Could you check a few things on this model? Use its own coordinates, in mm. Face numbers are marked on the shaded views. Give positions to 0.01 mm unless a question says otherwise; leave off trailing zeros. Order: outer loops, then holes, each group sorted by start corner. A loop starts at its lowest first (then second) coordinate and runs counter-clockwise, first axis right, second up. Notation, with made-up numbers: M -38,-15 L 15,-15 A18 ccw 15,8 Z; hole C -14,32 d8. An arc over 180 degrees is marked long. Answer in a Markdown table with one row per item. Add a question column.
```python
from build123d import *

# Parameters (mm, degrees)
F0_R     = 50
F0_R_2   = 8.25
F1_DEPTH = 22
F2_R     = 55
F3_DEPTH = 3


with BuildPart() as f1:
    # F0 (on Top) → F1 (new body)
    with BuildSketch(Plane.XY):
        Circle(F0_R)
        with BuildLine():
            Line((-33.445853, -33.728696), (-7.458661, -7.741504))
            ThreePointArc((-7.458661, -7.741504), (-5.97238, -8.938298), (-4.297911, -9.853449))
            Line((-4.297911, -9.853449), (-18.362078, -43.807352))
            ThreePointArc((-18.362078, -43.807352), (-26.389586, -39.494807), (-33.445853, -33.728696))
        make_face(mode=Mode.SUBTRACT)
        with BuildLine():
            ThreePointArc((-3.928359, -10.006523), (-2.097221, -10.543442), (-0.2, -10.748139))
            Line((-0.2, -10.748139), (-0.2, -47.499579))
            ThreePointArc((-0.2, -47.499579), (-9.26679, -46.587301), (-17.992526, -43.960425))
            Line((-17.992526, -43.960425), (-3.928359, -10.006523))
        make_face(mode=Mode.SUBTRACT)
        with BuildLine():
            ThreePointArc((-9.853449, -4.297911), (-8.938298, -5.97238), (-7.741504, -7.458661))
            Line((-7.741504, -7.458661), (-33.728696, -33.445853))
            ThreePointArc((-33.728696, -33.445853), (-39.494807, -26.389586), (-43.807352, -18.362078))
            Line((-43.807352, -18.362078), (-9.853449, -4.297911))
        make_face(mode=Mode.SUBTRACT)
        with BuildLine():
            Line((-47.499579, -0.2), (-10.748139, -0.2))
            ThreePointArc((-10.748139, -0.2), (-10.543442, -2.097221), (-10.006523, -3.928359))
            Line((-10.006523, -3.928359), (-43.960425, -17.992526))
            ThreePointArc((-43.960425, -17.992526), (-46.587301, -9.26679), (-47.499579, -0.2))
        make_face(mode=Mode.SUBTRACT)
        with BuildLine():
            Line((0.2, -47.499579), (0.2, -10.748139))
            ThreePointArc((0.2, -10.748139), (2.097221, -10.543442), (3.928359, -10.006523))
            Line((3.928359, -10.006523), (17.992526, -43.960425))
            ThreePointArc((17.992526, -43.960425), (9.26679, -46.587301), (0.2, -47.499579))
        make_face(mode=Mode.SUBTRACT)
        with BuildLine():
            ThreePointArc((4.297911, -9.853449), (5.97238, -8.938298), (7.458661, -7.741504))
            Line((7.458661, -7.741504), (33.445853, -33.728696))
            ThreePointArc((33.445853, -33.728696), (26.389586, -39.494807), (18.362078, -43.807352))
            Line((18.362078, -43.807352), (4.297911, -9.853449))
        make_face(mode=Mode.SUBTRACT)
        with BuildLine():
            Line((33.728696, -33.445853), (7.741504, -7.458661))
            ThreePointArc((7.741504, -7.458661), (8.938298, -5.97238), (9.853449, -4.297911))
            Line((9.853449, -4.297911), (43.807352, -18.362078))
            ThreePointArc((43.807352, -18.362078), (39.494807, -26.389586), (33.728696, -33.445853))
        make_face(mode=Mode.SUBTRACT)
        with BuildLine():
            ThreePointArc((10.006523, -3.928359), (10.543442, -2.097221), (10.748139, -0.2))
            Line((10.748139, -0.2), (47.499579, -0.2))
            ThreePointArc((47.499579, -0.2), (46.587301, -9.26679), (43.960425, -17.992526))
            Line((43.960425, -17.992526), (10.006523, -3.928359))
        make_face(mode=Mode.SUBTRACT)
        with BuildLine():
            ThreePointArc((-10.006523, 3.928359), (-10.543442, 2.097221), (-10.748139, 0.2))
            Line((-10.748139, 0.2), (-47.499579, 0.2))
            ThreePointArc((-47.499579, 0.2), (-46.587301, 9.26679), (-43.960425, 17.992526))
            Line((-43.960425, 17.992526), (-10.006523, 3.928359))
        make_face(mode=Mode.SUBTRACT)
        with BuildLine():
            Line((-33.728696, 33.445853), (-7.741504, 7.458661))
            ThreePointArc((-7.741504, 7.458661), (-8.938298, 5.97238), (-9.853449, 4.297911))
            Line((-9.853449, 4.297911), (-43.807352, 18.362078))
            ThreePointArc((-43.807352, 18.362078), (-39.494807, 26.389586), (-33.728696, 33.445853))
        make_face(mode=Mode.SUBTRACT)
        with BuildLine():
            ThreePointArc((-4.297911, 9.853449), (-5.97238, 8.938298), (-7.458661, 7.741504))
            Line((-7.458661, 7.741504), (-33.445853, 33.728696))
            ThreePointArc((-33.445853, 33.728696), (-26.389586, 39.494807), (-18.362078, 43.807352))
            Line((-18.362078, 43.807352), (-4.297911, 9.853449))
        make_face(mode=Mode.SUBTRACT)
        with BuildLine():
            ThreePointArc((-17.992526, 43.960425), (-9.26679, 46.587301), (-0.2, 47.499579))
            Line((-0.2, 47.499579), (-0.2, 10.748139))
            ThreePointArc((-0.2, 10.748139), (-2.097221, 10.543442), (-3.928359, 10.006523))
            Line((-3.928359, 10.006523), (-17.992526, 43.960425))
        make_face(mode=Mode.SUBTRACT)
        Circle(F0_R_2, mode=Mode.SUBTRACT)
        with BuildLine():
            Line((47.499579, 0.2), (10.748139, 0.2))
            ThreePointArc((10.748139, 0.2), (10.543442, 2.097221), (10.006523, 3.928359))
            Line((10.006523, 3.928359), (43.960425, 17.992526))
            ThreePointArc((43.960425, 17.992526), (46.587301, 9.26679), (47.499579, 0.2))
        make_face(mode=Mode.SUBTRACT)
        with BuildLine():
            ThreePointArc((9.853449, 4.297911), (8.938298, 5.97238), (7.741504, 7.458661))
            Line((7.741504, 7.458661), (33.728696, 33.445853))
            ThreePointArc((33.728696, 33.445853), (39.494807, 26.389586), (43.807352, 18.362078))
            Line((43.807352, 18.362078), (9.853449, 4.297911))
        make_face(mode=Mode.SUBTRACT)
        with BuildLine():
            ThreePointArc((3.928359, 10.006523), (2.097221, 10.543442), (0.2, 10.748139))
            Line((0.2, 10.748139), (0.2, 47.499579))
            ThreePointArc((0.2, 47.499579), (9.26679, 46.587301), (17.992526, 43.960425))
            Line((17.992526, 43.960425), (3.928359, 10.006523))
        make_face(mode=Mode.SUBTRACT)
        with BuildLine():
            Line((33.445853, 33.728696), (7.458661, 7.741504))
            ThreePointArc((7.458661, 7.741504), (5.97238, 8.938298), (4.297911, 9.853449))
            Line((4.297911, 9.853449), (18.362078, 43.807352))
            ThreePointArc((18.362078, 43.807352), (26.389586, 39.494807), (33.445853, 33.728696))
        make_face(mode=Mode.SUBTRACT)
    extrude(amount=F1_DEPTH)

    # F2 (on Top) → F3 (join)
    with BuildSketch(Plane.XY):
        Circle(F2_R)
    extrude(amount=-F3_DEPTH)


solid = f1.part
```
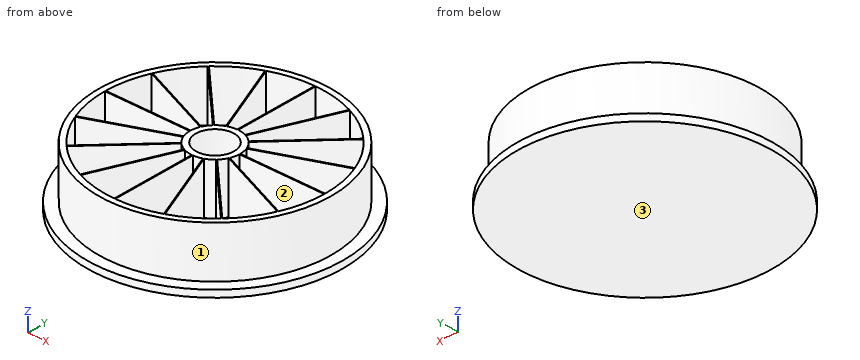
1. Suppose I cut it at A-A on x = 35. List the corners of the cut face in (y, z) for me.
2. Thinking about a two-plate mould opening in X: for the marked faces 1, 2 and 3, which applies, pulls with the +X half, pulls with the -X half, needs draft (parallel to the pull), parting line crosses it, or undercut?
3. Suppose I cut it at B-B on y = 37. List the corners of the cut face in (x, z) for me.
4. Will these pins go through, and if not, where does the flat tip stop? P1, Ø8, axis at x = 42.5, y = -31, coming from the +Z side; P2, Ø6, axis at y = 30.5, z = 17.5, coming from the +X side; P3, Ø6, axis at x = -25.5, y = 6, coming from the +Z side; P4, Ø11, axis at x = 33.5, z = 13.5, coming from the -Y side.
5. If I drill on line 1 along X through (y, z) = (-4, 11.5); line 2 along Y through (x, z) = (36.5, 13.25); line 3 along Y through (x, z) = (0, 7), over which ranges is the centre line in solid material (lowest first)? Write a range as [from, to].
6. Suppose I cut it at C-C on z = 3.5. Count the separate pieces of the cut face and the enclosed holes in it, plus the area to 3 significant figures.
Findings below:
| question | item | result |
|---|---|---|
| 1 | outline | M -42.43,-3 L 42.43,-3 L 42.43,0 L 35.71,0 L 35.71,22 L 32.11,22 L 32.11,0 L 14.71,0 L 14.71,22 L 14.28,22 L 14.28,0 L 0.2,0 L 0.2,22 L -0.2,22 L -0.2,0 L -14.28,0 L -14.28,22 L -14.71,22 L -14.71,0 L -32.11,0 L -32.11,22 L -35.71,22 L -35.71,0 L -42.43,0 Z |
| 2 | face 1 | parting line crosses it |
| 2 | face 2 | undercut |
| 2 | face 3 | needs draft |
| 3 | outline | M -40.69,-3 L 40.69,-3 L 40.69,0 L 33.63,0 L 33.63,22 L 29.79,22 L 29.79,0 L 15.54,0 L 15.54,22 L 15.11,22 L 15.11,0 L 0.2,0 L 0.2,22 L -0.2,22 L -0.2,0 L -15.11,0 L -15.11,22 L -15.54,22 L -15.54,0 L -29.79,0 L -29.79,22 L -33.63,22 L -33.63,0 L -40.69,0 Z |
| 4 | P1 | z = 22 |
| 4 | P2 | x = 41.76 |
| 4 | P3 | z = 0 |
| 4 | P4 | y = -41.42 |
| 5 | line 1 | [-49.84, -47.33], [-10.18, -7.22], [7.22, 10.18], [47.33, 49.84] |
| 5 | line 2 | [-34.17, -30.4], [-15.34, -14.9], [-0.2, 0.2], [14.9, 15.34], [30.4, 34.17] |
| 5 | line 3 | [-50, -8.25], [8.25, 50] |
| 6 | separate pieces | 1 |
| 6 | enclosed holes | 17 |
| 6 | area | 1,150 mm2 |
